Autodesk Inventor part; units mm, degrees
ref_plane "YZ Plane" through (0, 0, 0) normal (1, 0, 0) x (0, 1, 0)
ref_plane "XZ Plane" through (0, 0, 0) normal (0, 1, 0) x (-1, 0, 0)
ref_plane "XY Plane" through (0, 0, 0) normal (0, 0, 1) x (1, 0, 0)
sketch "Sketch1" plane through (0, 0, 0) normal (0, 1, 0) x (-1, 0, 0)
  line L0 (0, 0) -> (0, -152.4)
  line L1 (0, -152.4) -> (203.2, -152.4)
  line L2 (203.2, -152.4) -> (203.2, -31.75)
  line L3 (203.2, -31.75) -> (127, 0)
  line L4 (127, 0) -> (0, 0)
  dimension "d0" = 203.2
  dimension "d1" = 120.65
  dimension "d2" = 127
  dimension "d3" = 152.4
extrude "Extrusion1" add sketch "Sketch1" along normal blind 6.35
sketch "Sketch3" plane through (-127, 0, 0) normal (0, 0, 1) x (1, 0, 0)
  line L0 (0, 0) -> (127, 0)
  line L1 (127, 0) -> (127, 6.35)
  line L2 (0, 6.35) -> (127, 6.35)
  line L3 (0, 0) -> (0, 6.35)
extrude "Extrusion2" add sketch "Sketch3" along normal blind 71.12
sketch "Sketch4" plane through (-203.2, 0, -31.75) normal (-0.3846, 0, 0.9231) x (0.9231, 0, 0.3846)
  line L0 (0, 0) -> (82.55, 0)
  line L1 (82.55, 0) -> (82.55, 6.35)
  line L2 (0, 6.35) -> (82.55, 6.35)
  line L3 (0, 0) -> (0, 6.35)
  point P0 (199.7808, 0)
extrude "Extrusion3" add sketch "Sketch4" along normal blind 71.12
sketch "Sketch5" plane through (-203.2, 0, -152.4) normal (-1, 0, 0) x (0, 0, 1)
  line L0 (0, 0) -> (120.65, 0)
  line L1 (120.65, 0) -> (120.65, 6.35)
  line L2 (0, 6.35) -> (120.65, 6.35)
  line L3 (0, 0) -> (0, 6.35)
  point P0 (152.4, 0)
extrude "Extrusion4" add sketch "Sketch5" along normal blind 71.12
sketch "Sketch7" plane through (0, 6.35, 0) normal (0, 1, 0) x (1, 0, 0)
  line L0 (0, -71.12) -> (-127, -71.12)
  line L1 (-12.7, -71.12) -> (-19.05, -71.12)
  line L2 (-19.05, -71.12) -> (-19.05, -83.82)
  line L3 (-19.05, -83.82) -> (-12.7, -83.82)
  line L4 (-12.7, -83.82) -> (-12.7, -71.12)
  circle A0 centre (-15.875, -80.645) radius 1.397
  line L5 (0, 152.4) -> (0, -71.12)
  line L6 (-107.95, -71.12) -> (-114.3, -71.12)
  line L7 (-114.3, -71.12) -> (-114.3, -83.82)
  line L8 (-114.3, -83.82) -> (-107.95, -83.82)
  line L9 (-107.95, -83.82) -> (-107.95, -71.12)
  circle A1 centre (-111.125, -80.645) radius 1.397
  line L10 (-127, 0) -> (-127, -71.12)
  point P0 (0, 0)
  dimension "d13" = 12.7
  dimension "d14" = 6.35
  dimension "d15" = 2.794
  dimension "d16" = 3.175
  dimension "d17" = 12.7
  dimension "d18" = 3.175
  dimension "d19" = 12.7
  dimension "d20" = 6.35
  dimension "d21" = 2.794
  dimension "d22" = 3.175
  dimension "d23" = 3.175
  dimension "d24" = 0
  dimension "d25" = 12.7
extrude "Extrusion5" add sketch "Sketch7" against normal blind 6.35
sketch "Sketch8" plane through (0, 6.35, 0) normal (0, 1, 0) x (1, 0, 0)
  line L0 (-274.32, 152.4) -> (-274.32, 31.75)
  line L1 (-274.32, 44.45) -> (-287.02, 44.45)
  line L2 (-287.02, 44.45) -> (-287.02, 50.8)
  line L3 (-287.02, 50.8) -> (-274.32, 50.8)
  line L4 (-274.32, 50.8) -> (-274.32, 44.45)
  line L5 (-203.2, 31.75) -> (-274.32, 31.75)
  circle A0 centre (-283.845, 47.625) radius 1.397
  line L6 (-274.32, 133.35) -> (-287.02, 133.35)
  line L7 (-287.02, 133.35) -> (-287.02, 139.7)
  line L8 (-287.02, 139.7) -> (-274.32, 139.7)
  line L9 (-274.32, 139.7) -> (-274.32, 133.35)
  circle A1 centre (-283.845, 136.525) radius 1.397
  line L10 (0, 152.4) -> (-274.32, 152.4)
  point P0 (0, 0)
  point P1 (-272.7325, 33.3375)
  dimension "d33" = 6.35
  dimension "d34" = 12.7
  dimension "d35" = 12.7
  dimension "d36" = 2.794
  dimension "d37" = 3.175
  dimension "d38" = 3.175
  dimension "d39" = 6.35
  dimension "d40" = 12.7
  dimension "d41" = 2.794
  dimension "d42" = 3.175
  dimension "d43" = 3.175
  dimension "d44" = 0
  dimension "d45" = 12.7
extrude "Extrusion6" add sketch "Sketch8" against normal blind 6.35
sketch "Sketch9" plane through (0, 6.35, 0) normal (0, 1, 0) x (1, 0, 0)
  circle A0 centre (-38.1, 19.05) radius 1.397
  circle A1 centre (-63.5, 19.05) radius 1.397
  circle A2 centre (-38.1, 44.45) radius 1.397
  circle A3 centre (-63.5, 44.45) radius 1.397
  circle A4 centre (-127.2575, 106.1211) radius 1.397
  circle A5 centre (-152.6575, 106.1211) radius 1.397
  circle A6 centre (-127.2575, 131.5211) radius 1.397
  circle A7 centre (-152.6575, 131.5211) radius 1.397
  point P0 (0, 0)
  point P1 (-127, 0)
  dimension "d48" = 2.794
  dimension "d49" = 2.794
  dimension "d50" = 2.794
  dimension "d51" = 2.794
  dimension "d52" = 25.4
  dimension "d53" = 25.4
  dimension "d54" = 25.4
  dimension "d55" = 25.4
  dimension "d56" = 25.4
  dimension "d57" = 25.4
  dimension "d58" = 19.05
  dimension "d59" = 38.1
  dimension "d60" = 2.794
  dimension "d61" = 2.794
  dimension "d62" = 2.794
  dimension "d63" = 2.794
  dimension "d64" = 25.4
  dimension "d65" = 25.4
  dimension "d66" = 25.4
  dimension "d67" = 25.4
  dimension "d68" = 25.4
  dimension "d69" = 25.4
extrude "Extrusion7" cut sketch "Sketch9" against normal blind 6.35
sketch "Sketch10" plane through (0, 6.35, 0) normal (0, 1, 0) x (1, 0, 0)
  circle A0 centre (-9.271, 15.875) radius 1.524
  circle A1 centre (-9.271, 136.525) radius 1.524
  line L0 (0, 152.4) -> (-274.32, 152.4)
  circle A2 centre (-283.845, 47.625) radius 1.397
  circle A3 centre (-283.845, 136.525) radius 1.397
  line L1 (0, 152.4) -> (0, -71.12)
  circle A4 centre (-25.4, 143.129) radius 1.524
  circle A5 centre (-190.5, 143.129) radius 1.524
  point P0 (0, 0)
  point P1 (-203.2, 31.75)
  dimension "d72" = 3.048
  dimension "d73" = 3.048
  dimension "d74" = 15.875
  dimension "d75" = 120.65
  dimension "d76" = 9.271
  dimension "d77" = 9.271
  dimension "d78" = 3.048
  dimension "d79" = 3.048
  dimension "d80" = 9.271
  dimension "d81" = 25.4
  dimension "d82" = 12.7
  dimension "d83" = 9.271
  dimension "d101" = 88.9
extrude "Extrusion8" cut sketch "Sketch10" against normal blind 6.35 contours A0 | A1 | A4 | A5
sketch "Sketch11" plane through (0, 6.35, 0) normal (0, 1, 0) x (1, 0, 0)
  circle A0 centre (-178.7769, -16.9496) radius 8.763
  circle A1 centre (-107.95, -48.26) radius 4.2545
  circle A2 centre (-82.55, -35.56) radius 4.2545
  circle A3 centre (-107.95, -22.86) radius 4.2545
  line L0 (-19.05, -71.12) -> (-107.95, -71.12)
  line L1 (-127, 0) -> (-154.3538, -65.6492)
  line L2 (-127, 0) -> (-127, -71.12)
  line L3 (-154.3538, -65.6492) -> (-230.5538, -33.8992)
  point P0 (0, 0)
  dimension "d86" = 8.509
  dimension "d87" = 8.509
  dimension "d88" = 8.509
  dimension "d89" = 17.526
  dimension "d90" = 22.86
  dimension "d91" = 22.86
  dimension "d92" = 35.56
  dimension "d93" = 44.45
  dimension "d94" = 19.05
  dimension "d95" = 19.05
extrude "Extrusion9" cut sketch "Sketch11" against normal blind 6.35
sketch "Sketch12" plane through (0, 6.35, 0) normal (0, 1, 0) x (1, 0, 0)
  circle A0 centre (-36.1734, -35.56) radius 6.35
  line L0 (0, 152.4) -> (0, -71.12)
  line L1 (-127, 0) -> (-127, -71.12)
  point P0 (0, 0)
  dimension "d98" = 12.7
extrude "Extrusion10" cut sketch "Sketch12" against normal blind 6.35
sketch "Sketch13" plane through (0, 6.35, 0) normal (0, 1, 0) x (1, 0, 0)
  line L0 (0, 152.4) -> (-274.32, 152.4)
  line L1 (0, 152.4) -> (0, -71.12)
  circle A0 centre (-36.1734, -35.56) radius 6.35
  circle A1 centre (-107.95, -22.86) radius 4.2545
  circle A2 centre (-107.95, -48.26) radius 4.2545
  circle A3 centre (-82.55, -35.56) radius 4.2545
  circle A4 centre (-178.7769, -16.9496) radius 8.763
  circle A5 centre (-25.4, 143.129) radius 1.524
  circle A6 centre (-9.271, 15.875) radius 1.524
  circle A7 centre (-9.271, 136.525) radius 1.524
  circle A8 centre (-190.5, 143.129) radius 1.524
  circle A9 centre (-127.2575, 131.5211) radius 1.397
  circle A10 centre (-127.2575, 106.1211) radius 1.397
  circle A11 centre (-38.1, 44.45) radius 1.397
  circle A12 centre (-38.1, 19.05) radius 1.397
  circle A13 centre (-63.5, 19.05) radius 1.397
  circle A14 centre (-63.5, 44.45) radius 1.397
  circle A15 centre (-152.6575, 106.1211) radius 1.397
  circle A16 centre (-152.6575, 131.5211) radius 1.397
  circle A17 centre (-283.845, 47.625) radius 1.397
  circle A18 centre (-283.845, 136.525) radius 1.397
  circle A19 centre (-15.875, -80.645) radius 1.397
  circle A20 centre (-111.125, -80.645) radius 1.397
  line L2 (0, 152.4) -> (0, -71.12)
  line L3 (0, 152.4) -> (-274.32, 152.4)
  line L4 (-274.32, 139.7) -> (-274.32, 152.4)
  line L5 (-287.02, 139.7) -> (-274.32, 139.7)
  line L6 (-287.02, 133.35) -> (-287.02, 139.7)
  line L7 (-274.32, 133.35) -> (-287.02, 133.35)
  line L8 (-274.32, 50.8) -> (-274.32, 133.35)
  line L9 (-287.02, 50.8) -> (-274.32, 50.8)
  line L10 (-287.02, 44.45) -> (-287.02, 50.8)
  line L11 (-274.32, 44.45) -> (-287.02, 44.45)
  line L12 (-274.32, 31.75) -> (-274.32, 44.45)
  line L13 (-203.2, 31.75) -> (-274.32, 31.75)
  line L14 (-203.2, 31.75) -> (-230.5538, -33.8992)
  line L15 (-154.3538, -65.6492) -> (-230.5538, -33.8992)
  line L16 (-127, 0) -> (-154.3538, -65.6492)
  line L17 (-127, 0) -> (-127, -71.12)
  line L18 (-114.3, -71.12) -> (-127, -71.12)
  line L19 (-114.3, -71.12) -> (-114.3, -83.82)
  line L20 (-114.3, -83.82) -> (-107.95, -83.82)
  line L21 (-107.95, -83.82) -> (-107.95, -71.12)
  line L22 (-19.05, -71.12) -> (-107.95, -71.12)
  line L23 (-19.05, -71.12) -> (-19.05, -83.82)
  line L24 (-19.05, -83.82) -> (-12.7, -83.82)
  line L25 (-12.7, -83.82) -> (-12.7, -71.12)
  line L26 (0, -71.12) -> (-12.7, -71.12)
  point P0 (0, 0)
  dimension "d102" = 15.875
  dimension "d103" = 15.875
properties part number "Cut1"
Geometry check sheet. Reference: the model listing, model coordinates, mm. A direction names the side the tool comes from. Give positions to 0.01 mm unless a question says otherwise; leave off trailing zeros. Loops run counter-clockwise (first coordinate to the right, second up) from the corner with the lowest first, then second, coordinate; pieces in that order, holes last. Notation, with made-up numbers: (62.25, 0) -> (70.25, 0) arc R31 ccw to (70.25, 27) -> close; hole circle Ø1 at (-20.75, -13). An arc over 180 degrees is marked (long way). Answer in a Markdown table with one row per item. Add a question column.
1) Material ranges on probe 1 along Z at (x, y) = (-108, 5.75); probe 2 along X at (y, z) = (4.5, 33.5); probe 3 along X at (y, z) = (5.25, 22.86), recorded low to high. Write a range as from..to.
2) Cross-section at A-A on x = -82.55. Record the boundary of the cut face in (y, z).
3) Cross-section at B-B on z = 48.26. Record the boundary of the cut face in (x, y).
4) Cross-section at C-C on y = 5.25. State how many separate pieces and enclosed holes the cut face has, and give its area (3 significant figures).
5) Cross-section at D-D on x = -266.5. Record the boundary of the cut face in (y, z), and give its area (3 significant figures).
6) Set-up check for faces 1 (the face through (-281, 3, -44.45)), 2 (the face through (-281, 3, -139.7)), 3 (the face through (-64, 3, 71.12)), 4 (the face through (-281, 3, -133.35)): record each of +Z, -Z, +X, -X, +Y, -Y from which the full face is reachable in a straight line by a thin tool's end or side.
7) Draft check along X on faces 5 (the face through (-170.419, 3.219, 14.317)), 6 (the face through (-238, 3, -31.75)), 7 (the face through (-112.2, 3.2, 22.7)), 8 (the face through (-114.3, 3, 77)). Enter one of: pulls with the +X half, pulls with the -X half, needs draft (parallel to the pull), parting line crosses it, or undercut.
8) Gauge pin test, flat ends, axial feed: P1, Ø1.5, axis at x = -107, z = -12.5, coming from the -Y side; P2, Ø3, axis at y = 4, z = 74.5, coming from the -X side; P3, Ø3, axis at x = -279, y = 2, coming from the -Z side; P4, Ø3, axis at x = -8.5, y = 2, coming from the +Z side. Record the tip position at first contact, or that the pin passes through.
Outcome:
| question | item | result |
|---|---|---|
| 1 | probe 1 | z = -152.4..18.61, 27.11..44.01, 52.51..83.82 |
| 1 | probe 2 | x = -230.39..-140.96, -127..-86.27, -78.83..-42.18, -30.17..0 |
| 1 | probe 3 | x = -225.95..-185.25, -172.31..-136.52, -127..-112.2, -103.7..0 |
| 2 | outline | (0, -152.4) -> (6.35, -152.4) -> (6.35, 31.31) -> (0, 31.31) -> close; (0, 39.81) -> (6.35, 39.81) -> (6.35, 71.12) -> (0, 71.12) -> close |
| 3 | outline | (-196.09, 0) -> (-147.11, 0) -> (-147.11, 6.35) -> (-196.09, 6.35) -> close; (-127, 0) -> (-112.2, 0) -> (-112.2, 6.35) -> (-127, 6.35) -> close; (-103.7, 0) -> (0, 0) -> (0, 6.35) -> (-103.7, 6.35) -> close |
| 4 | separate pieces | 1 |
| 4 | enclosed holes | 21 |
| 4 | area | 52,900 mm^2 |
| 5 | outline | (0, -152.4) -> (6.35, -152.4) -> (6.35, -31.75) -> (0, -31.75) -> close |
| 5 | area | 766 mm^2 |
| 6 | face 1 | +Z, -X, +Y, -Y |
| 6 | face 2 | -Z, -X, +Y, -Y |
| 6 | face 3 | +Z, +Y, -Y |
| 6 | face 4 | -X, +Y, -Y |
| 7 | face 5 | undercut |
| 7 | face 6 | needs draft |
| 7 | face 7 | undercut |
| 7 | face 8 | pulls with the -X half |
| 8 | P1 | stops at y = 0 |
| 8 | P2 | stops at x = -114.3 |
| 8 | P3 | stops at z = -139.7 |
| 8 | P4 | stops at z = 71.12 |
